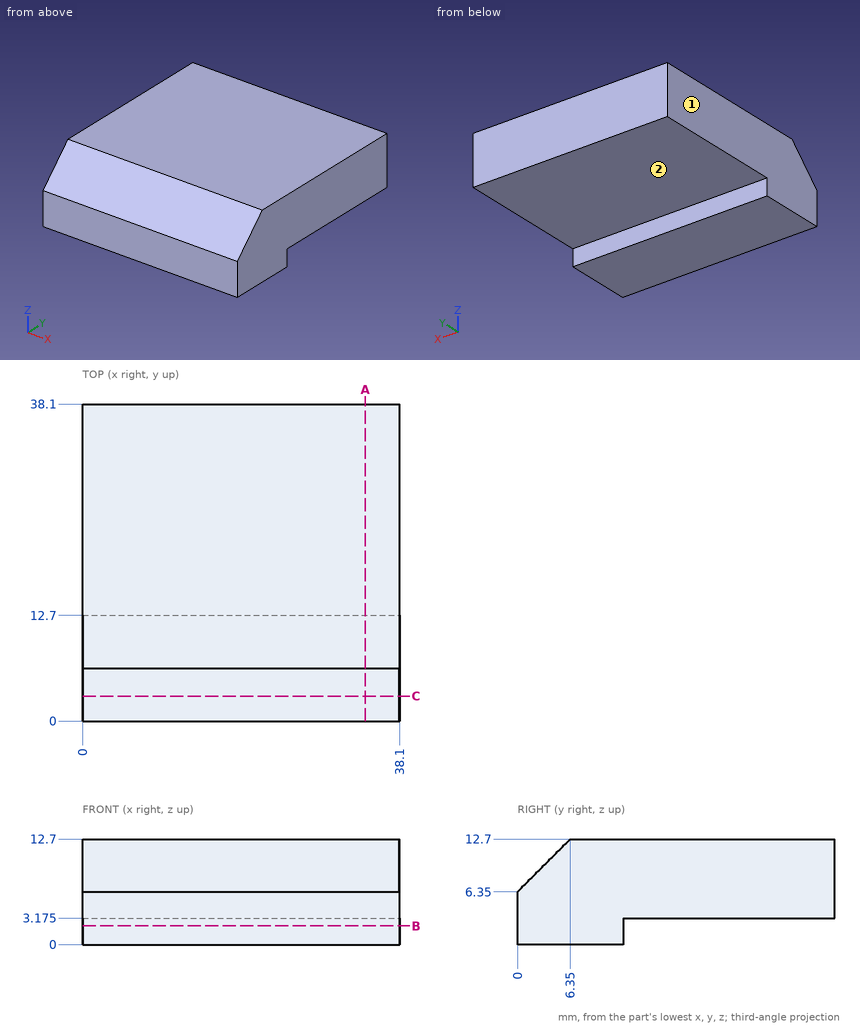
Answer from the drawing. Dimensions are ordinates in mm from the lowest x, y and z of the part. A direction names the side the tool comes from. Coordinates: 2 decimals unless noted, no trailing zeros. Order: outer loops, then holes, each group sorted by start corner. A loop starts at its lowest first (then second) coordinate and runs counter-clockwise, first axis right, second up. Notation, with made-up numbers: M -36.5,63 L -21.5,63 A36 ccw -21.5,102 Z; hole C 78,-9.5 d10. An arc over 180 degrees is marked long. Put each result on its own line as item: value. Start each with the question number.
Item 1: Section A-A, the plane x = 34 is taken. Determine the outline of the cut face in (y, z) (3 decimals).
Item 2: Consider probe 1 along Y at (x, z) = (16, 1); probe 2 along Z at (x, y) = (24.5, 30) (3 decimals); probe 3 along Y at (x, z) = (35.5, 8). Determine where each line is inside the solid, lowest interval first. Write a range as [from, to].
Item 3: Given pin 1 Ø5 at (y, z) = (18, 9.5) entering from -X; pin 2 Ø12.5 at (x, y) = (13.5, 29.5) entering from -Z (3 decimals); pin 3 Ø2.5 at (x, z) = (23, 1.5) entering from +Y, each flat-ended and moving along its own axis, determine where each tip first touches the part or whether it passes through.
Item 4: For the marked faces 1 and 2, determine the directions among +Z, -Z, +X, -X, +Y, -Y from which every point of the face is accessible in a straight line to the end or side of a thin tool.
Item 5: Section C-C, the plane y = 3 is taken. Determine the outline of the cut face in (x, z), plus the area to 3 significant figures.
Item 6: Section B-B, the plane z = 2.25 is taken. Determine the outline of the cut face in (x, y).
Computed:
1. outline: M 0,0 L 12.7,0 L 12.7,3.175 L 38.1,3.175 L 38.1,12.7 L 6.35,12.7 L 0,6.35 Z
2. probe 1: y = [0, 12.7]
2. probe 2: z = [3.175, 12.7]
2. probe 3: y = [1.65, 38.1]
3. pin 1: stops at x = 0
3. pin 2: stops at z = 3.175
3. pin 3: stops at y = 12.7
4. face 1: +Z, -Z, -X, +Y, -Y
4. face 2: -Z, +X, -X, +Y
5. outline: M 0,0 L 38.1,0 L 38.1,9.35 L 0,9.35 Z
5. area: 356 mm2
6. outline: M 0,0 L 38.1,0 L 38.1,12.7 L 0,12.7 Z
